Source: CAD feature listing. Evaluate the final solid. Frame: model axes, mm. A direction names the side the tool comes from. Round coordinates to 2 decimals unless told otherwise and drop trailing zeros. Order: outer loops, then holes, each group sorted by start corner. A loop starts at its lowest first (then second) coordinate and runs counter-clockwise, first axis right, second up.
```python
from build123d import *

# Parameters (mm, degrees)
F0_W     = 0.1980072791
F0_H     = 7.1694856525
F0_W_2   = 92.4687646329
F0_H_2   = 6.8283765789
F0_H_3   = 6.473645713
F0_H_4   = 5.7075782395
F0_H_5   = 7.0958843866
F0_H_6   = 7.2461878881
F0_H_7   = 6.6423406824
F1_DEPTH = 1.27


# Not quite as in the source:
# - a feature names something its author has since deleted; it is built from what else it names


with BuildPart() as f1:
    # F0 (on Front) → F1 (new body, symmetric)
    with BuildSketch(Plane.XZ):
        Polygon((-69.1910094554, 0), (-69.1910094554, -37.5021121278), (-69.0906792879, -37.5021121278), (-69.1058018093, -30.3326264753), (-69.1173589099, -24.8534827961), (-69.130230695, -18.7510560639), (-69.1435495608, -12.4366714017), (-69.1577431668, -5.7075782395), (-69.1697821021, 0), align=None)
        Polygon((-69.1058018093, -30.3326264753), (-69.0906792879, -37.5021121278), (68.9930021763, -37.5021121278), (68.9930021763, -30.3326264753), align=None)
        Polygon((-69.1910094554, 34.2864352491), (-69.1910094554, 0), (-69.1697821021, 0), (-23.4757624567, 0), (-23.4757624567, 6.473645713), (-23.4757624567, 13.1159863955), (-23.4757624567, 20.3621742836), (-23.4757624567, 27.4580586702), (-23.4757624567, 34.2864352491), align=None)
        with Locations((69.0920058158, -33.9173693016)):
            Rectangle(F0_W, F0_H)
        Polygon((68.9930021763, -25.3095924286), (68.9930021763, -30.3326264753), (69.1910094554, -30.3326264753), (69.1910094554, -25.3102463479), align=None)
        Polygon((-69.130230695, -18.7510560639), (-69.1173589099, -24.8534827961), (68.9930021763, -25.3095924286), (68.9930021763, -18.7510560639), align=None)
        with Locations((22.7586198598, 30.8722469596)):
            Rectangle(F0_W_2, F0_H_2)
        with Locations((22.7586198598, 3.2368228565)):
            Rectangle(F0_W_2, F0_H_3)
        Polygon((68.9930021763, -5.7075782395), (-69.1577431668, -5.7075782395), (-69.1435495608, -12.4366714017), (68.9930021763, -12.4186396162), align=None)
        Polygon((68.9930021763, -18.7510560639), (68.9930021763, -25.3095924286), (69.1910094554, -25.3102463479), (69.1910094554, -18.7510560639), align=None)
        with Locations((69.0920058158, 30.8722469596)):
            Rectangle(F0_W, F0_H_2)
        with Locations((69.0920058158, 3.2368228565)):
            Rectangle(F0_W, F0_H_3)
        with Locations((69.0920058158, -2.8537891197)):
            Rectangle(F0_W, F0_H_4)
        Polygon((69.1910094554, -5.7075782395), (68.9930021763, -5.7075782395), (68.9930021763, -12.4186396162), (69.1910094554, -12.4186137691), align=None)
        Polygon((68.9930021763, -12.4186396162), (68.9930021763, -18.7510560639), (69.1910094554, -18.7510560639), (69.1910094554, -12.4186137691), align=None)
        with Locations((69.0920058158, 23.9101164769)):
            Rectangle(F0_W, F0_H_5)
        with Locations((22.7586198598, 16.7390803395)):
            Rectangle(F0_W_2, F0_H_6)
        with Locations((69.0920058158, 9.7948160542)):
            Rectangle(F0_W, F0_H_7)
        with Locations((69.0920058158, 16.7390803395)):
            Rectangle(F0_W, F0_H_6)
    extrude(amount=F1_DEPTH, both=True)


solid = f1.part
```
1. Section D-D on x = -8.5. Return loops of the section in (y, z).
2. Section A-A on y = -0.3. Return loops of the section in (x, z), plus the area to 3 significant figures.
3. Access query for faces 3 (the face through (-1, 0, -37.502)), 4 (the face through (1, 0, -30.333)). Directions: +Z, -Z, +X, -X, +Y, -Y. A direction counts if a zero-diameter tool reaches every point of the face in a straight line with its end or side. Return the directions, or none.
4. Section B-B on z = 11. Return loops of the section in (x, y).
5. Pull-direction query (X, two-part tool) for faces 1 (the face through (1, 0, 34.286)), 2 (the face through (1, 0, -18.751)); classes: released by +X, released by -X, zero draft, split by the parting line, or undercut.
6. Line query: line 1 along Z through (x, y) = (-60.5, -0.7); line 2 along Z through (x, y) = (-6, 0.9); line 3 along Z through (x, y) = (-34, 1.1). Output: solid intervals per line, ascending.
7. Section C-C on x = -49.5. Return loops of the section in (y, z).
Result:
1. outline: (-1.27, -37.5) - (1.27, -37.5) - (1.27, -30.33) - (-1.27, -30.33) - close; (-1.27, -25.05) - (1.27, -25.05) - (1.27, -18.75) - (-1.27, -18.75) - close; (-1.27, -12.43) - (1.27, -12.43) - (1.27, -5.71) - (-1.27, -5.71) - close; (-1.27, 0) - (1.27, 0) - (1.27, 6.47) - (-1.27, 6.47) - close; (-1.27, 13.12) - (1.27, 13.12) - (1.27, 20.36) - (-1.27, 20.36) - close; (-1.27, 27.46) - (1.27, 27.46) - (1.27, 34.29) - (-1.27, 34.29) - close
2. outline: (-69.19, -37.5) - (69.19, -37.5) - (69.19, 34.29) - (-69.19, 34.29) - close; hole (-69.17, 0) - (-69.16, -5.71) - (68.99, -5.71) - (68.99, 0) - close; hole (-69.14, -12.44) - (-69.13, -18.75) - (68.99, -18.75) - (68.99, -12.42) - close; hole (-69.12, -24.85) - (-69.11, -30.33) - (68.99, -30.33) - (68.99, -25.31) - close; hole (-23.48, 6.47) - (68.99, 6.47) - (68.99, 13.12) - (-23.48, 13.12) - close; hole (-23.48, 20.36) - (68.99, 20.36) - (68.99, 27.46) - (-23.48, 27.46) - close
2. area: 6,280 mm2
3. face 3: -Z, +X, -X, +Y, -Y
3. face 4: +Y, -Y
4. outline: (-69.19, -1.27) - (-23.48, -1.27) - (-23.48, 1.27) - (-69.19, 1.27) - close; (68.99, -1.27) - (69.19, -1.27) - (69.19, 1.27) - (68.99, 1.27) - close
5. face 1: zero draft
5. face 2: undercut
6. line 1: z = -37.5 to -30.33, -24.88 to -18.75, -12.44 to -5.71, 0 to 34.29
6. line 2: z = -37.5 to -30.33, -25.06 to -18.75, -12.43 to -5.71, 0 to 6.47, 13.12 to 20.36, 27.46 to 34.29
6. line 3: z = -37.5 to -30.33, -24.97 to -18.75, -12.43 to -5.71, 0 to 34.29
7. outline: (-1.27, -37.5) - (1.27, -37.5) - (1.27, -30.33) - (-1.27, -30.33) - close; (-1.27, -24.92) - (1.27, -24.92) - (1.27, -18.75) - (-1.27, -18.75) - close; (-1.27, -12.43) - (1.27, -12.43) - (1.27, -5.71) - (-1.27, -5.71) - close; (-1.27, 0) - (1.27, 0) - (1.27, 34.29) - (-1.27, 34.29) - close
